The listing builds one solid part. Answer for the finished solid, in the listing's coordinates (mm). Round coordinates to 2 decimals unless told otherwise and drop trailing zeros. Order: outer loops, then holes, each group sorted by start corner. A loop starts at its lowest first (then second) coordinate and runs counter-clockwise, first axis right, second up. Notation, with made-up numbers: (-38.75, 6) -> (20.25, 6) arc R11 ccw to (20.25, 15) -> close; hole circle Ø5 at (-3, -9.75). An arc over 180 degrees is marked (long way). Return JSON: item names as keys, results as strings. Group by question number.
(1) Each of these flat-tipped pins is pushed along its axis until it touches: pin 1 (8.5 mm diameter, centred on x = 34, z = 12, fed in from -Y); pin 2 (1 mm diameter, centred on x = 63.5, z = 29.5, fed in from +Y); pin 3 (1 mm diameter, centred on y = 24.5, z = 29, fed in from -X); pin 4 (1 mm diameter, centred on x = 22, y = 10.5, fed in from -Z). Where does it stop, or does it pass through?
(2) The part is cut by section C-C (x = -12). Determine the outline of the cut face in (y, z).
(3) The part is cut by section D-D (y = 9). Determine the outline of the cut face in (x, z), plus the area to 3 significant figures.
(4) The part is cut by section B-B (y = 3). Determine the outline of the cut face in (x, z).
(5) Consider line 1 (X direction, y = 6, z = 16.5); line 2 (Y direction, x = 58, z = 28.25); line 3 (Y direction, x = -35.5, z = 9). Determine where each line is inside the solid, lowest interval first. Write a range as [from, to].
(6) The part is cut by section A-A (z = 9.75). Count the separate pieces of the cut face and the enclosed holes in it, plus the area to 3 significant figures.
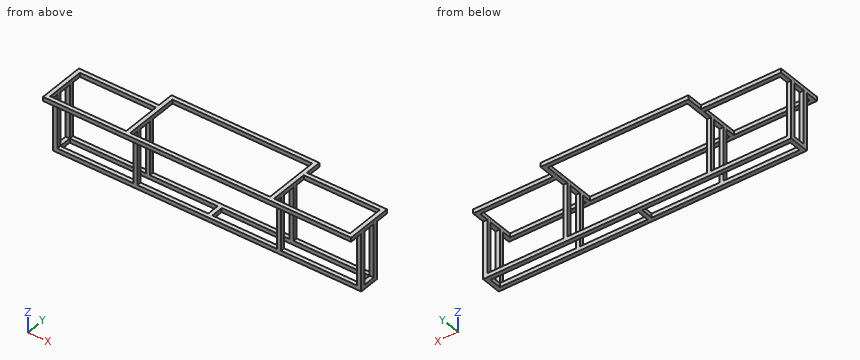
from build123d import *

# Parameters (mm, degrees)
F0_W     = 1.9999997169
F0_H     = 2
F0_H_2   = 6
F0_W_2   = 37.0000002831
F0_W_3   = 2
F1_DEPTH = 2
F2_DEPTH = 30
F3_START = 28
F0_H_3   = 4.5
F3_DEPTH = 2


with BuildPart() as f1:
    # F0 (on Top) → F1 (new body)
    with BuildSketch(Plane.XY):
        with Locations((-73.9999998584, 13.5)):
            Rectangle(F0_W, F0_H)
        with Locations((-73.9999998584, 9.5)):
            Rectangle(F0_W, F0_H_2)
        with Locations((-73.9999998584, 5.5)):
            Rectangle(F0_W, F0_H)
        with Locations((-54.4999998584, 5.5)):
            Rectangle(F0_W_2, F0_H)
        with Locations((-54.4999998584, 13.5)):
            Rectangle(F0_W_2, F0_H)
        with Locations((-34.9999998584, 13.5)):
            Rectangle(F0_W, F0_H)
        Polygon((-34, 14.5), (-34, 12.5), (-1, 12.5), (1, 12.5), (34, 12.5), (34, 14.5), align=None)
        with Locations((-34.9999998584, 5.5)):
            Rectangle(F0_W, F0_H)
        Polygon((-34, 6.5), (-34, 4.5), (34, 4.5), (34, 6.5), (1, 6.5), (-1, 6.5), align=None)
        with Locations((0, 9.5)):
            Rectangle(F0_W_3, F0_H_2)
        with Locations((34.9999998584, 13.5)):
            Rectangle(F0_W, F0_H)
        with Locations((34.9999998584, 5.5)):
            Rectangle(F0_W, F0_H)
        with Locations((54.4999998584, 5.5)):
            Rectangle(F0_W_2, F0_H)
        with Locations((54.4999998584, 13.5)):
            Rectangle(F0_W_2, F0_H)
        with Locations((73.9999998584, 13.5)):
            Rectangle(F0_W, F0_H)
        with Locations((73.9999998584, 9.5)):
            Rectangle(F0_W, F0_H_2)
        with Locations((73.9999998584, 5.5)):
            Rectangle(F0_W, F0_H)
    extrude(amount=F1_DEPTH)

    # F0 (on Top) → F2 (join)
    with BuildSketch(Plane.XY):
        with Locations((-73.9999998584, 5.5)):
            Rectangle(F0_W, F0_H)
        with Locations((-73.9999998584, 13.5)):
            Rectangle(F0_W, F0_H)
        with Locations((-34.9999998584, 5.5)):
            Rectangle(F0_W, F0_H)
        with Locations((-34.9999998584, 13.5)):
            Rectangle(F0_W, F0_H)
        with Locations((34.9999998584, 5.5)):
            Rectangle(F0_W, F0_H)
        with Locations((34.9999998584, 13.5)):
            Rectangle(F0_W, F0_H)
        with Locations((73.9999998584, 5.5)):
            Rectangle(F0_W, F0_H)
        with Locations((73.9999998584, 13.5)):
            Rectangle(F0_W, F0_H)
    extrude(amount=F2_DEPTH)

    # F0 (on Top) → F3 (join)
    with BuildSketch(Plane.XY.offset(F3_START)):
        Polygon((-74.9999997169, 14.5), (-73, 14.5), (-73, 19), (-35.9999997169, 19), (-35.9999997169, 20.9999997169), (-74.9999997169, 20.9999997169), align=None)
        Polygon((-35.9999997169, 0), (-73, 0), (-73, 4.5), (-74.9999997169, 4.5), (-74.9999997169, -1.9999997169), (74.9999997169, -1.9999997169), (74.9999997169, 4.5), (73, 4.5), (73, 0), (35.9999997169, 0), (34, 0), (-34, 0), align=None)
        with Locations((-34.9999998584, 2.25)):
            Rectangle(F0_W, F0_H_3)
        with Locations((-34.9999998584, 9.5)):
            Rectangle(F0_W, F0_H_2)
        with Locations((-34.9999998584, 16.75)):
            Rectangle(F0_W, F0_H_3)
        Polygon((-35.9999997169, 20.9999997169), (-35.9999997169, 19), (-34, 19), (-34, 27), (34, 27), (34, 19), (35.9999997169, 19), (35.9999997169, 20.9999997169), (35.9999997169, 28.9999997169), (-35.9999997169, 28.9999997169), align=None)
        with Locations((34.9999998584, 16.75)):
            Rectangle(F0_W, F0_H_3)
        Polygon((73, 14.5), (74.9999997169, 14.5), (74.9999997169, 20.9999997169), (35.9999997169, 20.9999997169), (35.9999997169, 19), (73, 19), align=None)
        with Locations((34.9999998584, 9.5)):
            Rectangle(F0_W, F0_H_2)
        with Locations((34.9999998584, 2.25)):
            Rectangle(F0_W, F0_H_3)
        with Locations((-34.9999998584, 5.5)):
            Rectangle(F0_W, F0_H)
        with Locations((-73.9999998584, 5.5)):
            Rectangle(F0_W, F0_H)
        with Locations((-73.9999998584, 9.5)):
            Rectangle(F0_W, F0_H_2)
        with Locations((-73.9999998584, 13.5)):
            Rectangle(F0_W, F0_H)
        with Locations((-34.9999998584, 13.5)):
            Rectangle(F0_W, F0_H)
        with Locations((34.9999998584, 13.5)):
            Rectangle(F0_W, F0_H)
        with Locations((34.9999998584, 5.5)):
            Rectangle(F0_W, F0_H)
        with Locations((73.9999998584, 5.5)):
            Rectangle(F0_W, F0_H)
        with Locations((73.9999998584, 9.5)):
            Rectangle(F0_W, F0_H_2)
        with Locations((73.9999998584, 13.5)):
            Rectangle(F0_W, F0_H)
    extrude(amount=F3_DEPTH)


solid = f1.part
Answer below:
{
 "1": {"pin 1": "stops at y = 4.5", "pin 2": "stops at y = 21", "pin 3": "stops at x = -36", "pin 4": "passes through"},
 "2": {"outline": "(-2, 28) -> (0, 28) -> (0, 30) -> (-2, 30) -> close; (4.5, 0) -> (6.5, 0) -> (6.5, 2) -> (4.5, 2) -> close; (12.5, 0) -> (14.5, 0) -> (14.5, 2) -> (12.5, 2) -> close; (27, 28) -> (29, 28) -> (29, 30) -> (27, 30) -> close"},
 "3": {"outline": "(-75, 0) -> (-73, 0) -> (-73, 2) -> (-75, 2) -> close; (-75, 28) -> (-73, 28) -> (-73, 30) -> (-75, 30) -> close; (-36, 28) -> (-34, 28) -> (-34, 30) -> (-36, 30) -> close; (-1, 0) -> (1, 0) -> (1, 2) -> (-1, 2) -> close; (34, 28) -> (36, 28) -> (36, 30) -> (34, 30) -> close; (73, 0) -> (75, 0) -> (75, 2) -> (73, 2) -> close; (73, 28) -> (75, 28) -> (75, 30) -> (73, 30) -> close", "area": "28.0 mm²"},
 "4": {"outline": "(-75, 28) -> (-73, 28) -> (-73, 30) -> (-75, 30) -> close; (-36, 28) -> (-34, 28) -> (-34, 30) -> (-36, 30) -> close; (34, 28) -> (36, 28) -> (36, 30) -> (34, 30) -> close; (73, 28) -> (75, 28) -> (75, 30) -> (73, 30) -> close"},
 "5": {"line 1": "x = [-75, -73], [-36, -34], [34, 36], [73, 75]", "line 2": "y = [-2, 0], [19, 21]", "line 3": "y = [4.5, 6.5], [12.5, 14.5]"},
 "6": {"separate pieces": "8", "enclosed holes": "0", "area": "32.0 mm²"}
}
